Design review of the part shown in the three views and the two pictorial views. Dimensions are in mm from the part's minimum x, y and z. Coordinates: 2 decimals unless noted, no trailing zeros. Loops run counter-clockwise (first coordinate to the right, second up) from the corner with the lowest first, then second, coordinate; pieces in that order, holes last. Notation, with made-up numbers: M 49,9.25 L 57,9.25 A20 cw 57,13.25 Z; hole C 48.25,80.5 d6. An arc over 180 degrees is marked long. Put each result on its own line as item: value. Start each with the question number.
(1) Take a section at B-B, the plane z = 6.75. Give the boundary of the cut face in (x, y).
(2) For probe 1 along Y at (x, z) = (25, 4); probe 2 along Y at (x, z) = (12, 9.25); probe 3 along X at (y, z) = (179.5, 4), list the stretches that pass through material, from the lowest coordinate up. Write a range as [from, to].
(3) Take a section at D-D, the plane x = 12. Give the boundary of the cut face in (y, z), then the cut area to 3 significant figures.
(4) Take a section at C-C, the plane x = 36. Give the boundary of the cut face in (y, z).
(5) Clearance check with flat-ended pins moving along their axes: pin 1 (2 mm diameter, centred on x = 13, z = 2, fed in from -Y); pin 2 (6 mm diameter, centred on x = 35.5, z = 4, fed in from +Y); pin 3 (4 mm diameter, centred on x = 28, z = 1.5, fed in from +Y). State where each tip first meets the part, or that it passes through.
(6) Take a section at A-A, the plane x = 25. Give the boundary of the cut face in (y, z).
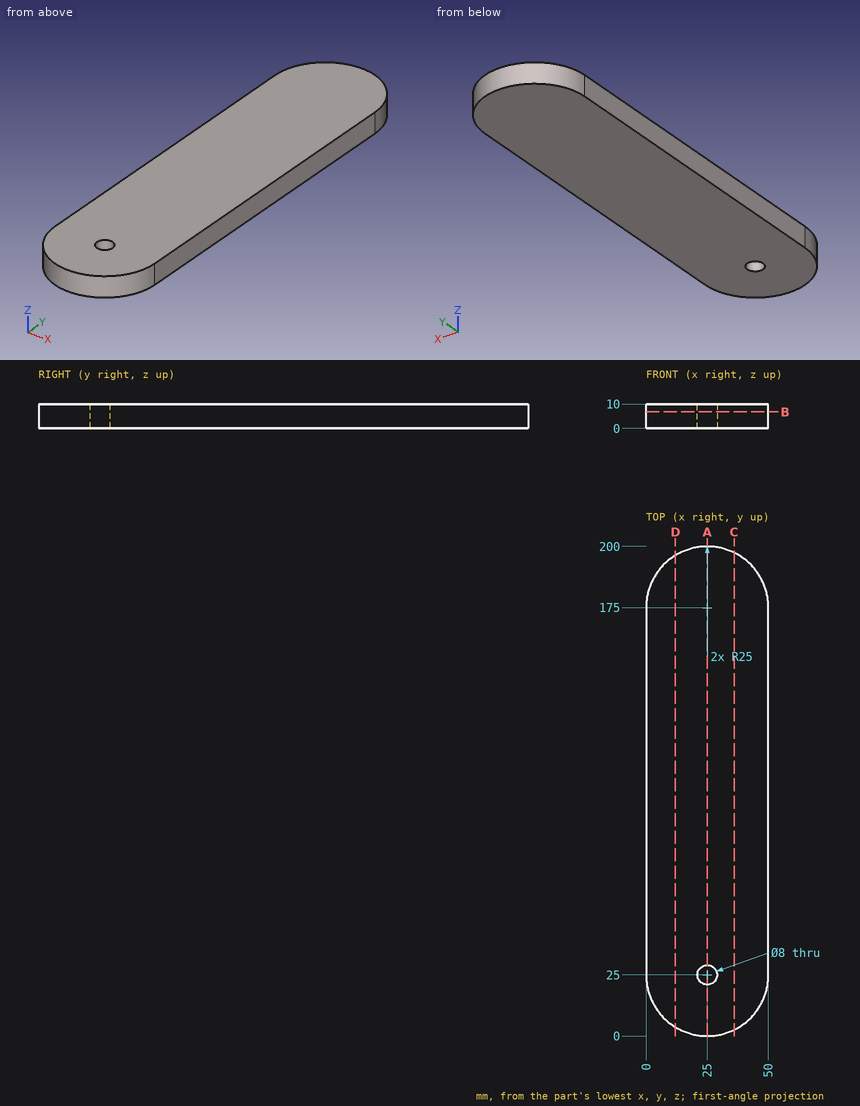
Computed values:
1. outline: M 0,25 A25 ccw 50,25 L 50,175 A25 ccw 0,175 Z; hole C 25,25 d8
2. probe 1: y = [0, 21], [29, 200]
2. probe 2: y = [3.65, 196.35]
2. probe 3: x = [0.41, 49.59]
3. outline: M 3.65,0 L 196.35,0 L 196.35,10 L 3.65,10 Z
3. area: 1,930 mm^2
4. outline: M 2.55,0 L 197.45,0 L 197.45,10 L 2.55,10 Z
5. pin 1: stops at y = 2.55
5. pin 2: stops at y = 198.85
5. pin 3: stops at y = 199.98
6. outline: M 0,0 L 21,0 L 21,10 L 0,10 Z; M 29,0 L 200,0 L 200,10 L 29,10 Z
